Geometry check sheet. Reference: the model listing, model coordinates, mm. Face numbers are marked on the shaded views. A direction names the side the tool comes from. Coordinates: 2 decimals unless noted, no trailing zeros. Write each loop counter-clockwise with the first axis right and the second up, starting at its lowest first coordinate (ties: lowest second). Pieces come first, ordered by that corner, then holes.
from build123d import *
from build123d.topology import SkipClean

# Parameters (mm, degrees)
BOSS_EXTRUDE1_DEPTH = 44.5
SKETCH2_W           = 6
SKETCH2_H           = 12
CUT_EXTRUDE1_DEPTH  = 10
BOSS_EXTRUDE2_DEPTH = 8.5
CUT_EXTRUDE2_DEPTH  = 11
SKETCH4_W           = 7
SKETCH4_H           = 8.5
BOSS_EXTRUDE3_DEPTH = 5
SKETCH5_R           = 1.25
CUT_EXTRUDE3_DEPTH  = 81.179486155
SKETCH7_R           = 1.25
CUT_EXTRUDE4_DEPTH  = 10
CUT_EXTRUDE6_DEPTH  = 3.5
BOSS_EXTRUDE4_DEPTH = 3


with BuildPart() as part:
    # Sketch1 → Boss-Extrude1 (new body)
    with BuildSketch(Plane(origin=(0, 0, 0), x_dir=(1, 0, 0), z_dir=(0, 1, 0))):
        Polygon((0, 0), (2, 0), (2, 6.5), (57, 6.5), (57, 0), (59, 0), (59, 8.5), (0, 8.5), align=None)
    extrude(amount=BOSS_EXTRUDE1_DEPTH)

    # Sketch2 → Cut-Extrude1 (cut)
    with BuildSketch(Plane(origin=(59, 0, 0), x_dir=(0, 0, -1), z_dir=(1, 0, 0))):
        with Locations((3, 29)):
            Rectangle(SKETCH2_W, SKETCH2_H)
    extrude(amount=-CUT_EXTRUDE1_DEPTH, mode=Mode.SUBTRACT)

    # Sketch3 → Boss-Extrude2 (add)
    with BuildSketch(Plane(origin=(0, 0, -8.5), x_dir=(-1, 0, 0), z_dir=(0, 0, -1))):
        with BuildLine():
            Line((-59, 6.145643924), (-59, 8))
            Line((-59, 8), (-59.5, 8))
            ThreePointArc((-59.5, 8), (-62.5, 5), (-59.5, 2))
            Line((-59.5, 2), (-59, 2))
            Line((-59, 2), (-59, 3.854356076))
            ThreePointArc((-59, 3.854356076), (-60.75, 5), (-59, 6.145643924))
        make_face()
        with BuildLine():
            Line((0.5, 8), (0, 8))
            Line((0, 8), (0, 6.145643924))
            ThreePointArc((0, 6.145643924), (1.184653197, 6.045825033), (1.75, 5))
            ThreePointArc((1.75, 5), (1.184653197, 3.954174967), (0, 3.854356076))
            Line((0, 3.854356076), (0, 2))
            Line((0, 2), (0.5, 2))
            ThreePointArc((0.5, 2), (3.5, 5), (0.5, 8))
        make_face()
    extrude(amount=-BOSS_EXTRUDE2_DEPTH)

    # Sketch3_3 → Cut-Extrude2 (cut)
    with SkipClean():  # the faces are left unmerged after this step: merging them gives an invalid solid
        with BuildSketch(Plane(origin=(0, 0, -8.5), x_dir=(-1, 0, 0), z_dir=(0, 0, -1))):
            with BuildLine():
                ThreePointArc((-58.25, 5), (-58.454174967, 5.684653197), (-59, 6.145643924))
                Line((-59, 6.145643924), (-59, 3.854356076))
                ThreePointArc((-59, 3.854356076), (-58.454174967, 4.315346803), (-58.25, 5))
            make_face()
            with BuildLine():
                Line((-59, 3.854356076), (-59, 6.145643924))
                ThreePointArc((-59, 6.145643924), (-60.75, 5), (-59, 3.854356076))
            make_face()
            with BuildLine():
                ThreePointArc((1.75, 5), (1.184653197, 6.045825033), (0, 6.145643924))
                Line((0, 6.145643924), (0, 3.854356076))
                ThreePointArc((0, 3.854356076), (1.184653197, 3.954174967), (1.75, 5))
            make_face()
            with BuildLine():
                Line((0, 3.854356076), (0, 6.145643924))
                ThreePointArc((0, 6.145643924), (-0.75, 5), (0, 3.854356076))
            make_face()
        extrude(amount=-CUT_EXTRUDE2_DEPTH, mode=Mode.SUBTRACT)

    # Sketch4 → Boss-Extrude3 (add)
    with SkipClean():  # the faces are left unmerged after this step: merging them gives an invalid solid
        with BuildSketch(Plane(origin=(0, 44.5, 0), x_dir=(1, 0, 0), z_dir=(0, 1, 0))):
            with Locations((3.5, 4.25)):
                Rectangle(SKETCH4_W, SKETCH4_H)
            with Locations((55.5, 4.25)):
                Rectangle(SKETCH4_W, SKETCH4_H)
        extrude(amount=BOSS_EXTRUDE3_DEPTH)

    # Sketch5 → Cut-Extrude3 (cut, through all)
    with SkipClean():  # the faces are left unmerged after this step: merging them gives an invalid solid
        with BuildSketch(Plane(origin=(0, 0, -8.5), x_dir=(-1, 0, 0), z_dir=(0, 0, -1))):
            with Locations((-55.5, 47)):
                Circle(SKETCH5_R)
            with Locations((-3.5, 47)):
                Circle(SKETCH5_R)
        extrude(amount=-CUT_EXTRUDE3_DEPTH, mode=Mode.SUBTRACT)

    # Sketch7 → Cut-Extrude4 (cut)
    with SkipClean():  # the faces are left unmerged after this step: merging them gives an invalid solid
        with BuildSketch(Plane(origin=(0, 0, -8.5), x_dir=(-1, 0, 0), z_dir=(0, 0, -1))):
            with Locations((-53.6, 2.9)):
                Circle(SKETCH7_R)
            with Locations((-5.4, 2.9)):
                Circle(SKETCH7_R)
            with Locations((-53.6, 40.95)):
                Circle(SKETCH7_R)
            with Locations((-5.4, 40.95)):
                Circle(SKETCH7_R)
        extrude(amount=-CUT_EXTRUDE4_DEPTH, mode=Mode.SUBTRACT)

    # Sketch3_4 → Cut-Extrude6 (cut)
    with SkipClean():  # the faces are left unmerged after this step: merging them gives an invalid solid
        with BuildSketch(Plane(origin=(0, 0, -8.5), x_dir=(-1, 0, 0), z_dir=(0, 0, -1))):
            with BuildLine():
                Line((-59, 6.145643924), (-59, 8))
                Line((-59, 8), (-59.5, 8))
                ThreePointArc((-59.5, 8), (-62.5, 5), (-59.5, 2))
                Line((-59.5, 2), (-59, 2))
                Line((-59, 2), (-59, 3.854356076))
                ThreePointArc((-59, 3.854356076), (-60.75, 5), (-59, 6.145643924))
            make_face()
            with BuildLine():
                Line((0.5, 8), (0, 8))
                Line((0, 8), (0, 6.145643924))
                ThreePointArc((0, 6.145643924), (1.184653197, 6.045825033), (1.75, 5))
                ThreePointArc((1.75, 5), (1.184653197, 3.954174967), (0, 3.854356076))
                Line((0, 3.854356076), (0, 2))
                Line((0, 2), (0.5, 2))
                ThreePointArc((0.5, 2), (3.5, 5), (0.5, 8))
            make_face()
        extrude(amount=-CUT_EXTRUDE6_DEPTH, mode=Mode.SUBTRACT)

    # Sketch3_5 → Boss-Extrude4 (add)
    with SkipClean():  # the faces are left unmerged after this step: merging them gives an invalid solid
        with BuildSketch(Plane(origin=(0, 0, -8.5), x_dir=(-1, 0, 0), z_dir=(0, 0, -1))):
            with BuildLine():
                Line((0, 3.854356076), (0, 6.145643924))
                ThreePointArc((0, 6.145643924), (-0.75, 5), (0, 3.854356076))
            make_face()
            with BuildLine():
                ThreePointArc((-58.25, 5), (-58.454174967, 5.684653197), (-59, 6.145643924))
                Line((-59, 6.145643924), (-59, 3.854356076))
                ThreePointArc((-59, 3.854356076), (-58.454174967, 4.315346803), (-58.25, 5))
            make_face()
        extrude(amount=-BOSS_EXTRUDE4_DEPTH)


solid = part.part
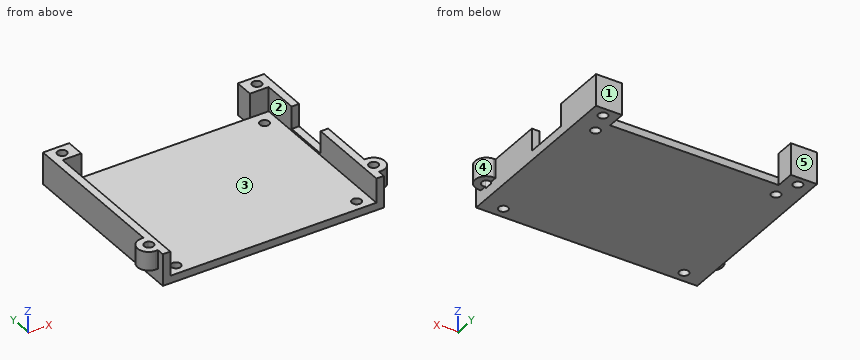
1. Access from +Z, -Z, +X, -X, +Y, -Y to the whole of each face (thin tool, end or side, straight path). Record for the marked faces 1 and 2.
Computed values:
face 1: +Z, -Z, +X, -X, +Y
face 2: +Z, -Y
2. Sectioned sample at D-D, the plane y = 47. Record the boundary of the cut face in (x, z).
Computed values:
outline: (0, -8.5) - (2.25, -8.5) - (2.25, 0) - (0, 0) - close; (4.75, -8.5) - (7, -8.5) - (7, 0) - (4.75, 0) - close; (52, -8.5) - (54.25, -8.5) - (54.25, 0) - (52, 0) - close; (56.75, -8.5) - (59, -8.5) - (59, 0) - (56.75, 0) - close
3. Thickness scan on line 1 along Y through (x, z) = (5.4, -7.15); line 2 along Y through (x, z) = (55.5, -6); line 3 along X through (y, z) = (43.5, -4.5). Record the ranges inside material, lowest first.
Computed values:
line 1: y = 0 to 1.65, 4.15 to 39.7, 42.2 to 49.5
line 2: y = 44.5 to 45.75, 48.25 to 49.5
line 3: x = 0 to 2, 57 to 59
4. Sectioned sample at C-C, the plane x = 5.5. Record the boundary of the cut face in (y, z), and give its area (3 significant figures).
Computed values:
outline: (0, -8.5) - (1.65, -8.5) - (1.65, -6.5) - (0, -6.5) - close; (4.15, -8.5) - (39.7, -8.5) - (39.7, -6.5) - (4.15, -6.5) - close; (42.2, -8.5) - (49.5, -8.5) - (49.5, 0) - (44.5, 0) - (44.5, -6.5) - (42.2, -6.5) - close
area: 122 mm2
5. Gauge pin test, flat ends, axial feed: pin 1 Ø2 at (x, y) = (53.6, 40.95) entering from -Z; pin 2 Ø1.5 at (y, z) = (18.5, -6.5) entering from -X; pin 3 Ø22 at (x, y) = (23.5, 23) entering from +Z; pin 4 Ø4 at (y, z) = (14.5, -5.5) entering from +X. Record the tip position at first contact, or that the pin passes through.
Computed values:
pin 1: passes through
pin 2: stops at x = 0
pin 3: stops at z = -6.5
pin 4: stops at x = 59
6. Sectioned sample at A-A, the plane z = -1.25. Record the boundary of the cut face in (x, y).
Computed values:
outline: (-0.5, 2) - (0, 2) - (0, 0) - (2, 0) - (2, 44.5) - (7, 44.5) - (7, 49.5) - (0, 49.5) - (0, 8) - (-0.5, 8) arc R3 ccw to start; (52, 44.5) - (57, 44.5) - (57, 35) - (59, 35) - (59, 49.5) - (52, 49.5) - close; (57, 0) - (59, 0) - (59, 2) - (59.5, 2) arc R3 ccw to (59.5, 8) - (59, 8) - (59, 23) - (57, 23) - close; hole circle Ø2.5 at (-0.5, 5); hole circle Ø2.5 at (3.5, 47); hole circle Ø2.5 at (55.5, 47); hole circle Ø2.5 at (59.5, 5)
7. Sectioned sample at B-B, the plane y = 40.95. Record the boundary of the cut face in (x, z), and give its area (3 significant figures).
Computed values:
outline: (0, -8.5) - (4.15, -8.5) - (4.15, -6.5) - (2, -6.5) - (2, 0) - (0, 0) - close; (6.65, -8.5) - (52.35, -8.5) - (52.35, -6.5) - (6.65, -6.5) - close; (54.85, -8.5) - (59, -8.5) - (59, 0) - (57, 0) - (57, -6.5) - (54.85, -6.5) - close
area: 134 mm2
8. Draft check along X on the marked faces 3, 4 and 5. Enter one of: released by +X, released by -X, zero draft, split by the parting line, or undercut.
Computed values:
face 3: undercut
face 4: released by +X
face 5: zero draft
